Build history of the part. All positions in model axes, mm. A direction names the side the tool comes from. Give positions to 0.01 mm unless a question says otherwise; leave off trailing zeros. Loops run counter-clockwise (first coordinate to the right, second up) from the corner with the lowest first, then second, coordinate; pieces in that order, holes last. Notation, with made-up numbers: M 44.5,84 L 98.5,84 A10 ccw 98.5,102 Z; hole C 53.5,24.25 d9. An arc over 180 degrees is marked long. Answer as a JSON object with one key per item and string values. Group by question number.
1. Slice it at B-B (x = 13.5). List the corners of the cut face in (y, z), then the cut area to 3 significant figures.
2. Drill centre lines: line 1 along Y through (x, z) = (32, 2.35); line 2 along X through (y, z) = (28, 2); line 3 along Y through (x, z) = (1, 1.7). Where is each one in solid material? Low to high. Write a range as [from, to].
3. Slice it at A-A (y = 30). List the corners of the cut face in (x, z).
4. Mould opens along X. For faces 1 (the face through (-5.413, -8.443, 1.417)), 2 (the face through (44.482, 19, 1)), 3 (the face through (19, 38.354, 1)) say: released by +X, released by -X, zero draft, split by the parting line, or undercut.
5. Slice it at C-C (z = 1.05). List the corners of the cut face in (x, y) (3 decimals).
6. 3-axis set-ups, long thin cutter, end or side, ignore diameter. For faces 4 (the face through (37.493, 0.687, 1.377)), 5 (the face through (19, 47.752, 1)): which of +Z, -Z, +X, -X, +Y, -Y reach the whole face in a straight line?
Autodesk Inventor part; units mm, degrees
ref_plane "YZ Plane" through (0, 0, 0) normal (1, 0, 0) x (0, 1, 0)
ref_plane "XZ Plane" through (0, 0, 0) normal (0, 1, 0) x (-1, 0, 0)
ref_plane "XY Plane" through (0, 0, 0) normal (0, 0, 1) x (1, 0, 0)
sketch "Sketch1" plane through (0, 0, 0) normal (0, 0, 1) x (1, 0, 0)
  line L0 (0, 19.177) -> (19.0817, 19.177)
  line L1 (-6.3183, -9.398) -> (44.4817, -9.398)
  line L2 (44.4817, -9.398) -> (44.4817, 47.752)
  line L3 (44.4817, 47.752) -> (-6.3183, 47.752)
  line L4 (-6.3183, 47.752) -> (-6.3183, -9.398)
  line L5 (-6.3183, -9.398) -> (44.4817, 47.752) construction
  line L6 (44.4817, -9.398) -> (-6.3183, 47.752) construction
  line L7 (2.305, 0) -> (35.8584, 0)
  line L8 (38.1444, 2.286) -> (38.1444, 36.068)
  line L9 (35.8584, 38.354) -> (2.305, 38.354)
  line L10 (0.019, 36.068) -> (0.019, 2.286)
  line L11 (0.019, 0) -> (38.1444, 38.354) construction
  line L12 (38.1444, 0) -> (0.019, 38.354) construction
  arc A0 (2.305, 38.354) -> (0.019, 36.068) centre (2.305, 36.068) ccw
  arc A1 (38.1444, 36.068) -> (35.8584, 38.354) centre (35.8584, 36.068) ccw
  arc A2 (35.8584, 0) -> (38.1444, 2.286) centre (35.8584, 2.286) ccw
  arc A3 (0.019, 2.286) -> (2.305, 0) centre (2.305, 2.286) ccw
  dimension "d15" = 50.8
  dimension "d16" = 57.15
  dimension "d19" = 38.1254
  dimension "d20" = 38.354
  dimension "d21" = 2.286
extrude "Extrusion1" add sketch "Sketch1" along normal blind 2.794
fillet "Fillet4" radius 3.175 4 edges at (-6.3183, 47.752, 1.397) (44.4817, 47.752, 1.397) (44.4817, -9.398, 1.397) (-6.3183, -9.398, 1.397)
properties part number "ESC Hole Test"
Established:
{
 "1": {"outline": "M -9.4,0 L 0,0 L 0,2.79 L -9.4,2.79 Z; M 38.35,0 L 47.75,0 L 47.75,2.79 L 38.35,2.79 Z", "area": "52.5 mm^2"},
 "2": {"line 1": "y = [-9.4, 0], [38.35, 47.75]", "line 2": "x = [-6.32, 0.02], [38.14, 44.48]", "line 3": "y = [-9.4, 0.41], [37.94, 47.75]"},
 "3": {"outline": "M -6.32,0 L 0.02,0 L 0.02,2.79 L -6.32,2.79 Z; M 38.14,0 L 44.48,0 L 44.48,2.79 L 38.14,2.79 Z"},
 "4": {"face 1": "released by -X", "face 2": "released by +X", "face 3": "undercut"},
 "5": {"outline": "M -6.318,-6.223 A3.175 ccw -3.143,-9.398 L 41.307,-9.398 A3.175 ccw 44.482,-6.223 L 44.482,44.577 A3.175 ccw 41.307,47.752 L -3.143,47.752 A3.175 ccw -6.318,44.577 Z; hole M 0.019,2.286 A2.286 ccw 2.305,0 L 35.858,0 A2.286 ccw 38.144,2.286 L 38.144,36.068 A2.286 ccw 35.858,38.354 L 2.305,38.354 A2.286 ccw 0.019,36.068 Z"},
 "6": {"face 4": "+Z, -Z", "face 5": "+Z, -Z, +X, -X, +Y"}
}
